```python
from build123d import *

# Parameters (mm, degrees)
SKETCH1_R           = 10
SKETCH1_R_2         = 4.5
BOSS_EXTRUDE1_DEPTH = 20
SKETCH2_R           = 6.625
CUT_EXTRUDE1_DEPTH  = 13
SKETCH3_R           = 6.625
CUT_EXTRUDE2_DEPTH  = 5


with BuildPart() as part:
    # Sketch1 → Boss-Extrude1 (new body)
    with BuildSketch(Plane(origin=(0, 0, 0), x_dir=(1, 0, 0), z_dir=(0, 1, 0))):
        Circle(SKETCH1_R)
        Circle(SKETCH1_R_2, mode=Mode.SUBTRACT)
    extrude(amount=BOSS_EXTRUDE1_DEPTH)

    # Sketch2 → Cut-Extrude1 (cut)
    with BuildSketch(Plane(origin=(0, 20, 0), x_dir=(1, 0, 0), z_dir=(0, 1, 0))):
        Circle(SKETCH2_R)
    extrude(amount=-CUT_EXTRUDE1_DEPTH, mode=Mode.SUBTRACT)

    # Sketch3 → Cut-Extrude2 (cut)
    with BuildSketch(Plane.XZ):
        Circle(SKETCH3_R)
    extrude(amount=-CUT_EXTRUDE2_DEPTH, mode=Mode.SUBTRACT)


solid = part.part
```
The listing builds one solid part. Answer for the finished solid, in the listing's coordinates (mm). A direction names the side the tool comes from. Coordinates: 2 decimals unless noted, no trailing zeros. Loops run counter-clockwise (first coordinate to the right, second up) from the corner with the lowest first, then second, coordinate; pieces in that order, holes last. Notation, with made-up numbers: M 34,59 L 70,59 A22 cw 70,91 Z; hole C 40.5,86.5 d7. An arc over 180 degrees is marked long. Answer as a JSON object with one key per item and string values. Group by question number.
Item 1: Section C-C (y = 8.25) is taken. Write down the section's boundary in (x, z) (3 decimals), and give its area (3 significant figures).
Item 2: Determine the mould class of faces 4 (the face through (0, 7, -5)), 5 (the face through (0, 5, 5)), 6 (the face through (-2.17, 9.86, 9.76)), 7 (the face through (7, 0, 2)) for opening direction Z: +Z half, -Z half, draft (parallel to the pull), parting line (faces both ways), or undercut.
Item 3: Section B-B (x = 0) is taken. Write down the section's boundary in (y, z) (3 decimals), and give its area (4 significant figures).
Item 4: Consider L1, parallel to X at y = 16, z = 0 (3 decimals); L2, parallel to Z at x = 3.75, y = 6. Determine where each line is inside the solid, lowest interval first.
Item 5: Each of these flat-tipped pins is pushed along its axis until it touches: P1, Ø8, axis at y = 6, z = 7, coming from the -X side; P2, Ø8, axis at x = 7.5, y = 17.5, coming from the +Z side; P3, Ø2, axis at x = 2, y = 14, coming from the -Z side. Where does it stop, or does it pass through?
Item 6: Which of the six approach directions +Z, -Z, +X, -X, +Y, -Y give full straight-line access (tool end or side, diameter ignored) to faces 1 (the face through (-0.59, 5.99, -4.46)), 2 (the face through (3.562, 2.465, 5.586)), 3 (the face through (3.562, 13.591, -5.586))?
Item 7: Section A-A (z = 0) is taken. Write down the section's boundary in (x, y) (3 decimals).
Item 8: Section D-D (x = -7.75) is taken. Write down the section's boundary in (y, z).
Solved:
{
 "1": {"outline": "C 0,0 d20; hole C 0,0 d13.25", "area": "176 mm2"},
 "2": {"face 4": "undercut", "face 5": "undercut", "face 6": "parting line", "face 7": "draft"},
 "3": {"outline": "M 0,-10 L 20,-10 L 20,-6.625 L 7,-6.625 L 7,-4.5 L 5,-4.5 L 5,-6.625 L 0,-6.625 Z; M 0,6.625 L 5,6.625 L 5,4.5 L 7,4.5 L 7,6.625 L 20,6.625 L 20,10 L 0,10 Z", "area": "143.5 mm2"},
 "4": {"L1": "x = -10 to -6.625, 6.625 to 10", "L2": "z = -9.27 to -2.49, 2.49 to 9.27"},
 "5": {"P1": "stops at x = -9.54", "P2": "stops at z = 9.37", "P3": "stops at z = -9.95"},
 "6": {"face 1": "+Y, -Y", "face 2": "-Y", "face 3": "+Y"},
 "7": {"outline": "M -10,0 L -6.625,0 L -6.625,5 L -4.5,5 L -4.5,7 L -6.625,7 L -6.625,20 L -10,20 Z; M 4.5,5 L 6.625,5 L 6.625,0 L 10,0 L 10,20 L 6.625,20 L 6.625,7 L 4.5,7 Z"},
 "8": {"outline": "M 0,-6.32 L 20,-6.32 L 20,6.32 L 0,6.32 Z"}
}
